Verification items for the finished model (mm, model axes). A direction names the side the tool comes from. Round coordinates to 2 decimals unless told otherwise and drop trailing zeros. Order: outer loops, then holes, each group sorted by start corner. A loop starts at its lowest first (then second) coordinate and runs counter-clockwise, first axis right, second up.
```python
from build123d import *

# Parameters (mm, degrees)
SKETCH1_W           = 150
SKETCH1_H           = 150
BOSS_EXTRUDE1_DEPTH = 100
SKETCH5_R           = 70
CUT_EXTRUDE2_DEPTH  = 100
SKETCH6_R           = 100
BOSS_EXTRUDE4_DEPTH = 10
SKETCH7_W           = 100
SKETCH7_H           = 100
CUT_EXTRUDE3_DEPTH  = 100


with BuildPart() as part:
    # Sketch1 → Boss-Extrude1 (new body)
    with BuildSketch(Plane(origin=(0, 0, 0), x_dir=(1, 0, 0), z_dir=(0, 1, 0))):
        with BuildLine():
            Line((363.145565834, 275.992438563), (363.145565834, 275.741810419))
            ThreePointArc((363.145565834, 275.741810419), (198.145565834, 225.992438563), (363.145565834, 176.243066708))
            Line((363.145565834, 176.243066708), (563.145565834, 176.243066708))
            Line((563.145565834, 176.243066708), (563.145565834, 275.741810419))
            Line((563.145565834, 275.741810419), (563.145565834, 275.992438563))
            Line((563.145565834, 275.992438563), (363.145565834, 275.992438563))
        make_face()
        with Locations((638.145565834, 226.117752636)):
            Rectangle(SKETCH1_W, SKETCH1_H)
    extrude(amount=BOSS_EXTRUDE1_DEPTH)

    # Sketch5 → Cut-Extrude2 (cut)
    with BuildSketch(Plane(origin=(0, 100, 0), x_dir=(1, 0, 0), z_dir=(0, 1, 0))):
        with Locations(Location((288.145565834, 225.992438563, 0), (0, 0, 270))):
            Circle(SKETCH5_R)
    extrude(amount=-CUT_EXTRUDE2_DEPTH, mode=Mode.SUBTRACT)

    # Sketch6 → Boss-Extrude4 (add)
    with BuildSketch(Plane(origin=(0, 100, 0), x_dir=(1, 0, 0), z_dir=(0, 1, 0))):
        with Locations(Location((288.145565834, 225.992438563, 0), (0, 0, 30))):
            Circle(SKETCH6_R)
    extrude(amount=BOSS_EXTRUDE4_DEPTH)

    # Sketch7 → Cut-Extrude3 (cut)
    with BuildSketch(Plane(origin=(0, 100, 0), x_dir=(1, 0, 0), z_dir=(0, 1, 0))):
        with Locations((638.145565834, 226.117752636)):
            Rectangle(SKETCH7_W, SKETCH7_H)
    extrude(amount=-CUT_EXTRUDE3_DEPTH, mode=Mode.SUBTRACT)


solid = part.part
```
1) Sectioned sample at B-B on y = 65. Record the cut outline in (x, z), then the cut area to 3 significant figures.
2) Sectioned sample at D-D on z = -167. Record the cut outline in (x, y), then the cut area to 3 significant figures.
3) Tool access check on faces 4 (the flat face through (637, 51, -176.118)), 5 (the flat face through (563.146, 49, -288)), 6 (the flat face through (637, 49, -301.118)), 7 (the cylindrical face through (219.81, 50.7, -241.17)), 8 (the flat face through (637, 49, -151.118)). Record the directions out of +Z, -Z, +X, -X, +Y, -Y that give a thin tool (end or side, any length) a straight path to the whole face; none if there is none.
4) Scan lines: probe 1 along X at (y, z) = (25, -228); probe 2 along Z at (x, y) = (599.5, 68); probe 3 along X at (y, z) = (53.5, -165). Record each from-to range of solid material in increasing order.
5) Sectioned sample at C-C on x = 272. Record the cut outline in (y, z) (1 decimal).
6) Go/stop test with flat-tipped pins: pin 1 Ø12 at (x, z) = (286.5, -212) entering from -Y; pin 2 Ø2 at (x, z) = (493, -254) entering from +Y; pin 3 Ø6 at (x, y) = (440.5, 97.5) entering from +Z. Record where each tip stops, or that it passes through.
7) Draft check along X on faces 1 (the flat face through (452, 0, -227)), 2 (the flat face through (713.146, 49, -225)), 3 (the flat face through (588.146, 51, -225)). Enter one of: released by +X, released by -X, zero draft, split by the parting line, or undercut.
8) Sectioned sample at A-A on z = -191. Record the cut outline in (x, y), then the cut area to 3 significant figures.
Returned:
1. outline: (363.15, -275.99) - (563.15, -275.99) - (563.15, -301.12) - (713.15, -301.12) - (713.15, -151.12) - (563.15, -151.12) - (563.15, -176.24) - (363.15, -176.24) arc R90 ccw (long way) to (363.15, -275.74) - close; hole circle Ø140 at (288.15, -225.99); hole (588.15, -276.12) - (688.15, -276.12) - (688.15, -176.12) - (588.15, -176.12) - close
1. area: 41,500 mm2
2. outline: (207.4, 100) - (220.18, 100) - (220.18, 0) - (250.46, 0) - (250.46, 100) - (325.83, 100) - (325.83, 0) - (356.12, 0) - (356.12, 100) - (368.89, 100) - (368.89, 110) - (207.4, 110) - close; (563.15, 0) - (713.15, 0) - (713.15, 100) - (563.15, 100) - close
2. area: 22,700 mm2
3. face 4: +Y, -Y
3. face 5: -Z, +Y, -Y
3. face 6: -Z, +X, +Y, -Y
3. face 7: -Y
3. face 8: +Z, +X, +Y, -Y
4. probe 1: x = 198.17 to 218.17, 358.12 to 588.15, 688.15 to 713.15
4. probe 2: z = -301.12 to -276.12, -176.12 to -151.12
4. probe 3: x = 221.96 to 253.8, 322.5 to 354.33, 563.15 to 713.15
5. outline: (0, -314.5) - (100, -314.5) - (100, -324.7) - (110, -324.7) - (110, -127.3) - (100, -127.3) - (100, -137.5) - (0, -137.5) - (0, -157.9) - (100, -157.9) - (100, -294.1) - (0, -294.1) - close
6. pin 1: stops at y = 100
6. pin 2: stops at y = 100
6. pin 3: stops at z = -176.24
7. face 1: zero draft
7. face 2: released by +X
7. face 3: undercut
8. outline: (194.47, 100) - (205.23, 100) - (205.23, 0) - (227.52, 0) - (227.52, 100) - (348.77, 100) - (348.77, 0) - (588.15, 0) - (588.15, 100) - (381.82, 100) - (381.82, 110) - (194.47, 110) - close; (688.15, 0) - (713.15, 0) - (713.15, 100) - (688.15, 100) - close
8. area: 30,500 mm2
